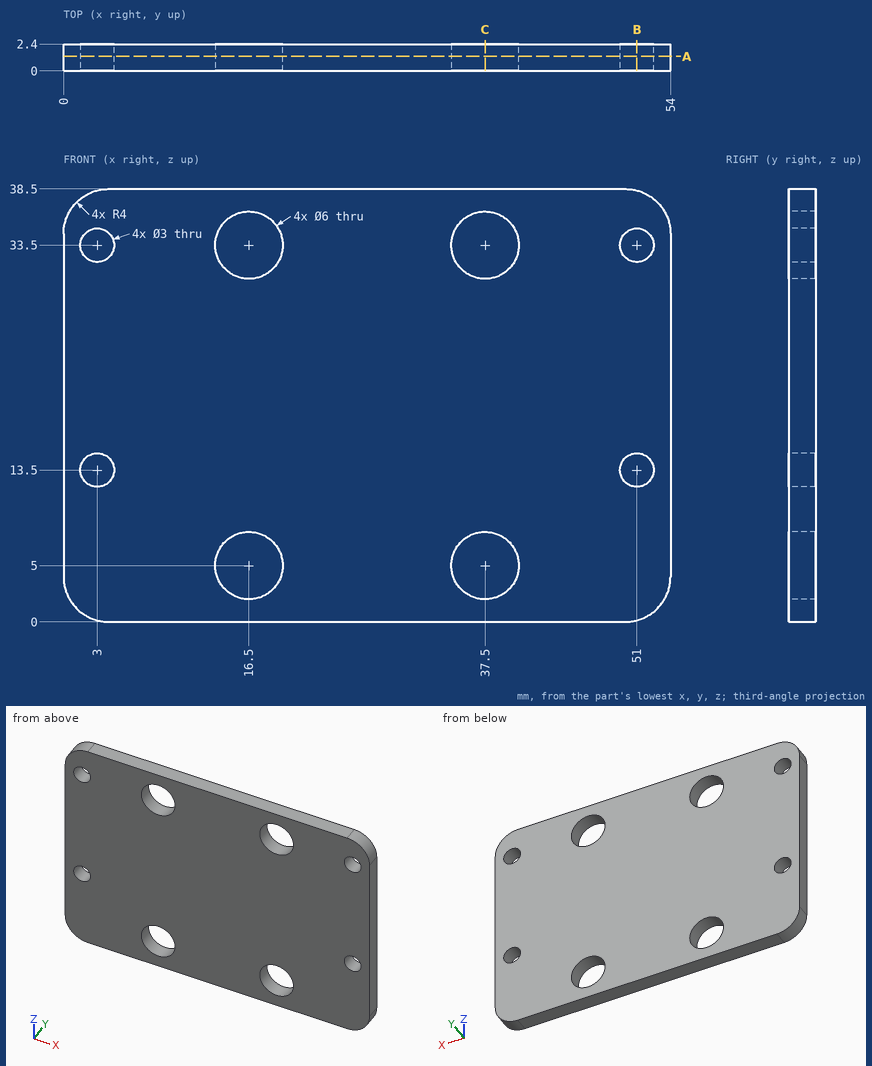
Job drawing, mm, ordinate dimensions from the low corner. One solid piece. Give positions to 0.01 mm unless a question says otherwise; leave off trailing zeros. Write each loop counter-clockwise with the first axis right and the second up, starting at its lowest first coordinate (ties: lowest second). Pieces come first, ordered by that corner, then holes. Notation, with made-up numbers: (46, 68) - (78, 68) arc R21 ccw to (78, 97) - close; hole circle Ø6 at (65, 54.5). An arc over 180 degrees is marked (long way). Use one line per item in the form item = value. Start each with the question number.
1. Drop a flat-ended pin along its axis: pin 1 Ø5.5 at (x, z) = (37.5, 5) entering from -Y. Give the stop position or say it passes through.
2. Band-saw the part on A-A on y = 1.3. Count the separate pieces of the cut face and the enclosed holes in it, plus the area to 3 significant figures.
3. Probe line 1 (X direction, y = 0.8, z = 13.5); line 2 (Z direction, x = 37.5, y = 0.6); line 3 (Z direction, x = 4, y = 0.9). List the from-to ranges inside material, lowest first. Write a range as [from, to].
4. Band-saw the part on B-B on x = 51. Write the cut outline in (y, z).
5. Band-saw the part on C-C on x = 37.5. Write the cut outline in (y, z), plus the area to 3 significant figures.
Conclusion:
q1.pin_1 = through
q2.separate_pieces = 1
q2.enclosed_holes = 8
q2.area = 1,920 mm²
q3.line_1 = [0, 1.5], [4.5, 49.5], [52.5, 54]
q3.line_2 = [0, 2], [8, 30.5], [36.5, 38.5]
q3.line_3 = [0, 12.38], [14.62, 32.38], [34.62, 38.5]
q4.outline = (0, 0.13) - (2.4, 0.13) - (2.4, 12) - (0, 12) - close; (0, 15) - (2.4, 15) - (2.4, 32) - (0, 32) - close; (0, 35) - (2.4, 35) - (2.4, 38.37) - (0, 38.37) - close
q5.outline = (0, 0) - (2.4, 0) - (2.4, 2) - (0, 2) - close; (0, 8) - (2.4, 8) - (2.4, 30.5) - (0, 30.5) - close; (0, 36.5) - (2.4, 36.5) - (2.4, 38.5) - (0, 38.5) - close
q5.area = 63.6 mm²
